Geometry check sheet. Reference: the model listing, model coordinates, mm. Face numbers are marked on the shaded views. A direction names the side the tool comes from. Coordinates: 2 decimals unless noted, no trailing zeros. Write each loop counter-clockwise with the first axis right and the second up, starting at its lowest first coordinate (ties: lowest second). Pieces come first, ordered by that corner, then holes.
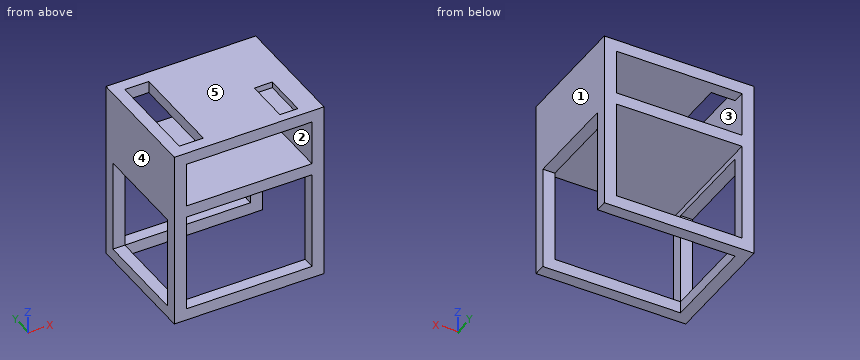
from build123d import *

# Parameters (mm, degrees)
F0_W      = 500
F0_H      = 600
F1_DEPTH  = 400
F3_W      = 80
F3_H      = 320
F4_DEPTH  = 200
F5_W      = 420
F5_H      = 520
F6_DEPTH  = 400
F7_W      = 400
F7_H      = 40
F8_DEPTH  = 420
F9_W      = 60
F9_H      = 150
F10_DEPTH = 20
F11_W     = 320
F11_H     = 350
F12_DEPTH = 625
F13_W     = 40
F13_H     = 40
F14_DEPTH = 325


with BuildPart() as f1:
    # F0 (on Front) → F1 (new body)
    with BuildSketch(Plane.XZ):
        with Locations((250, 300)):
            Rectangle(F0_W, F0_H)
    extrude(amount=F1_DEPTH)

    # F3 (on face) → F4 (cut)
    with BuildSketch(Plane.XY.offset(600)):
        with Locations((80, -200)):
            Rectangle(F3_W, F3_H)
    extrude(amount=-F4_DEPTH, mode=Mode.SUBTRACT)

    # F5 (on face) → F6 (cut)
    with BuildSketch(Plane.XZ.offset(400)):
        with Locations((250, 300)):
            Rectangle(F5_W, F5_H)
    extrude(amount=-F6_DEPTH, mode=Mode.SUBTRACT)

    # F7 (on face) → F8 (join)
    with BuildSketch(Plane(origin=(460, 0, 0), x_dir=(0, -1, 0), z_dir=(-1, 0, 0))):
        with Locations((200, 390)):
            Rectangle(F7_W, F7_H)
    extrude(amount=F8_DEPTH)

    # F9 (on face) → F10 (cut)
    with BuildSketch(Plane.XY.offset(600)):
        with Locations((400, -295)):
            Rectangle(F9_W, F9_H)
    extrude(amount=-F10_DEPTH, mode=Mode.SUBTRACT)

    # F11 (on face) → F12 (cut)
    with BuildSketch(Plane.YZ.offset(500)):
        with Locations((-200, 175)):
            Rectangle(F11_W, F11_H)
    extrude(amount=-F12_DEPTH, mode=Mode.SUBTRACT)

    # F13 (on face) → F14 (join)
    with BuildSketch(Plane.XZ.offset(40)):
        with Locations((20, 20)):
            Rectangle(F13_W, F13_H)
    extrude(amount=F14_DEPTH)


solid = f1.part
1. Thickness scan on line 1 along Z through (x, y) = (451, -362); line 2 along Z through (x, y) = (198, -84); line 3 along X through (y, z) = (-154.5, 547). Record the ranges inside material, lowest first.
Computed values:
line 1: z = 0 to 40, 370 to 410, 560 to 600
line 2: z = 370 to 410, 560 to 600
line 3: x = 0 to 40, 460 to 500
2. Draft check along Z on the marked faces 3, 4 and 5. Enter one of: released by +Z, released by -Z, zero draft, split by the parting line, or undercut.
Computed values:
face 3: undercut
face 4: zero draft
face 5: released by +Z
3. Sectioned sample at C-C, the plane z = 455.5. Record the boundary of the cut face in (x, y).
Computed values:
outline: (0, -400) - (40, -400) - (40, 0) - (0, 0) - close; (460, -400) - (500, -400) - (500, 0) - (460, 0) - close
4. Access from +Z, -Z, +X, -X, +Y, -Y to the whole of each face (thin tool, end or side, straight path). Record for the marked faces 1 and 2.
Computed values:
face 1: +Z, -Z, +X, +Y, -Y
face 2: +Y, -Y
5. Sectioned sample at D-D, the plane x = 93.5. Record the boundary of the cut face in (y, z), and give its area (3 significant figures).
Computed values:
outline: (-400, 0) - (-360, 0) - (-360, 40) - (-400, 40) - close; (-400, 370) - (0, 370) - (0, 410) - (-400, 410) - close; (-400, 560) - (-360, 560) - (-360, 600) - (-400, 600) - close; (-40, 0) - (0, 0) - (0, 40) - (-40, 40) - close; (-40, 560) - (0, 560) - (0, 600) - (-40, 600) - close
area: 22,400 mm2
6. Sectioned sample at B-B, the plane z = 80.5. Record the boundary of the cut face in (x, y), and give its area (3 significant figures).
Computed values:
outline: (0, -400) - (40, -400) - (40, -360) - (0, -360) - close; (0, -40) - (40, -40) - (40, 0) - (0, 0) - close; (460, -400) - (500, -400) - (500, -360) - (460, -360) - close; (460, -40) - (500, -40) - (500, 0) - (460, 0) - close
area: 6,400 mm2
7. Sectioned sample at A-A, the plane y = -264.5. Record the boundary of the cut face in (x, z), and give its area (3 significant figures).
Computed values:
outline: (0, 0) - (40, 0) - (40, 40) - (0, 40) - close; (0, 350) - (40, 350) - (40, 370) - (460, 370) - (460, 350) - (500, 350) - (500, 600) - (430, 600) - (430, 580) - (370, 580) - (370, 600) - (120, 600) - (120, 560) - (460, 560) - (460, 410) - (40, 410) - (40, 600) - (0, 600) - close
area: 50,800 mm2
8. Gauge pin test, flat ends, axial feed: pin 1 Ø1 at (x, y) = (236, -133) entering from -Z; pin 2 Ø12 at (x, y) = (74, -153) entering from +Z. Record the tip position at first contact, or that the pin passes through.
Computed values:
pin 1: stops at z = 370
pin 2: stops at z = 410
